Build history of the part. All positions in model axes, mm. A direction names the side the tool comes from. Give positions to 0.01 mm unless a question says otherwise; leave off trailing zeros. Order: outer loops, then holes, each group sorted by start corner. A loop starts at its lowest first (then second) coordinate and runs counter-clockwise, first axis right, second up. Notation, with made-up numbers: (37.25, 57) - (89.25, 57) arc R31 ccw to (89.25, 82) - close; hole circle Ø3 at (50.25, -34). An arc over 180 degrees is marked (long way). One line per item, written item: value.
```python
from build123d import *

# Parameters (mm, degrees)
SKETCH1_R               = 42.0875
BOSS_EXTRUDE1_DEPTH     = 24
SKETCH2_R               = 38.2875
CUT_EXTRUDE1_DEPTH      = 11
SKETCH3_R               = 34.2875
CUT_EXTRUDE2_DEPTH      = 10
SKETCH5_R               = 12.5
CUT_EXTRUDE4_DEPTH      = 1
CUT_EXTRUDE4_DEPTH_BACK = 25
CUT_EXTRUDE3_START      = -4
SKETCH4_R               = 1.5
CUT_EXTRUDE3_DEPTH      = 26
CIRPATTERN1_COUNT       = 4


with BuildPart() as part:
    # Sketch1 → Boss-Extrude1 (new body)
    with BuildSketch(Plane.XY.offset(-8)):
        Circle(SKETCH1_R)
    extrude(amount=BOSS_EXTRUDE1_DEPTH)

    # Sketch2 → Cut-Extrude1 (cut)
    with BuildSketch(Plane(origin=(0, 0, -8), x_dir=(-1, 0, 0), z_dir=(0, 0, -1))):
        Circle(SKETCH2_R)
    extrude(amount=-CUT_EXTRUDE1_DEPTH, mode=Mode.SUBTRACT)

    # Sketch3 → Cut-Extrude2 (cut)
    with BuildSketch(Plane(origin=(0, 0, 3), x_dir=(-1, 0, 0), z_dir=(0, 0, -1))):
        Circle(SKETCH3_R)
    extrude(amount=-CUT_EXTRUDE2_DEPTH, mode=Mode.SUBTRACT)

    # Sketch5 → Cut-Extrude4 (cut, two sides)
    with BuildSketch(Plane.XY.offset(16)) as cut_extrude4_sk:
        Circle(SKETCH5_R)
    extrude(amount=CUT_EXTRUDE4_DEPTH, mode=Mode.SUBTRACT)
    extrude(cut_extrude4_sk.sketch, amount=-CUT_EXTRUDE4_DEPTH_BACK, mode=Mode.SUBTRACT)

    # Sketch4 → Cut-Extrude3 (cut)
    with BuildSketch(Plane(origin=(0, 0, 13), x_dir=(-1, 0, 0), z_dir=(0, 0, -1)).offset(CUT_EXTRUDE3_START)):
        with Locations((-16.5, 0)):
            Circle(SKETCH4_R)
    cut_extrude3 = extrude(amount=CUT_EXTRUDE3_DEPTH, mode=Mode.SUBTRACT)

    # CirPattern1: Cut-Extrude3 ×4 about axis
    cirpattern1_axis = Axis((0, 0, 0), (0, 0, 1))
    for i in range(1, CIRPATTERN1_COUNT):
        add(cut_extrude3.rotate(cirpattern1_axis, i * 360 / CIRPATTERN1_COUNT), mode=Mode.SUBTRACT)


solid = part.part
```
(1) Pin check, flat tips, straight feed: P1, Ø10, axis at x = -1.5, y = 26, coming from the -Z side; P2, Ø1, axis at y = 2, z = -1.5, coming from the -X side; P3, Ø8, axis at y = -25.5, z = 5, coming from the -X side. Stop position of each tip, or through.
Completed:
P1: z = 13
P2: x = -42.06
P3: x = -36.18
(2) Slice it at D-D, the plane y = 32. Give the cut face in (x, z).
Completed:
outline: (-27.34, -8) - (-21.02, -8) - (-21.02, 3) - (-12.31, 3) - (-12.31, 13) - (12.31, 13) - (12.31, 3) - (21.02, 3) - (21.02, -8) - (27.34, -8) - (27.34, 16) - (-27.34, 16) - close
(3) Drill centre lines: line 1 (Y direction, x = 0, z = 8); line 2 (Z direction, x = 15, y = -12); line 3 (X direction, y = -5, z = 2.75). Where is each one in solid material? Low to high.
Completed:
line 1: -42.09 to -34.29, 34.29 to 42.09
line 2: 13 to 16
line 3: -41.79 to -37.96, 37.96 to 41.79
(4) Pull direction X, two halves, no side cores. Call faces 1 (the face through (19, -34, -8)), 2 (the face through (18, 0, 15)), 3 (the face through (40.144, 12.642, 3.832)): +X half, -X half, draft (parallel to the pull), parting line (faces both ways), or undercut.
Completed:
face 1: draft
face 2: undercut
face 3: parting line
(5) Slice it at A-A, the plane x = 0. Give the cut face in (y, z), and give its area (3 significant figures).
Completed:
outline: (-42.09, -8) - (-38.29, -8) - (-38.29, 3) - (-34.29, 3) - (-34.29, 13) - (-18, 13) - (-18, 16) - (-42.09, 16) - close; (-15, 13) - (-12.5, 13) - (-12.5, 16) - (-15, 16) - close; (12.5, 13) - (15, 13) - (15, 16) - (12.5, 16) - close; (18, 13) - (34.29, 13) - (34.29, 3) - (38.29, 3) - (38.29, -8) - (42.09, -8) - (42.09, 16) - (18, 16) - close
area: 399 mm²
(6) Slice it at C-C, the plane x = 10. Give the cut face in (y, z), and give its area (3 significant figures).
Completed:
outline: (-40.88, -8) - (-36.96, -8) - (-36.96, 3) - (-32.8, 3) - (-32.8, 13) - (-7.5, 13) - (-7.5, 16) - (-40.88, 16) - close; (7.5, 13) - (32.8, 13) - (32.8, 3) - (36.96, 3) - (36.96, -8) - (40.88, -8) - (40.88, 16) - (7.5, 16) - close
area: 448 mm²
(7) Slice it at B-B, the plane y = 11. Give the cut face in (x, z), and give its area (3 significant figures).
Completed:
outline: (-40.62, -8) - (-36.67, -8) - (-36.67, 3) - (-32.48, 3) - (-32.48, 13) - (-5.94, 13) - (-5.94, 16) - (-40.62, 16) - close; (5.94, 13) - (32.48, 13) - (32.48, 3) - (36.67, 3) - (36.67, -8) - (40.62, -8) - (40.62, 16) - (5.94, 16) - close
area: 458 mm²
(8) 3-axis set-ups, long thin cutter, end or side, ignore diameter. For faces 4 (the face through (4.984, 37.962, -2.577)), 5 (the face through (-18, 0, 15)): which of +Z, -Z, +X, -X, +Y, -Y reach the whole face in a straight line?
Completed:
face 4: -Z
face 5: +Z, -Z
